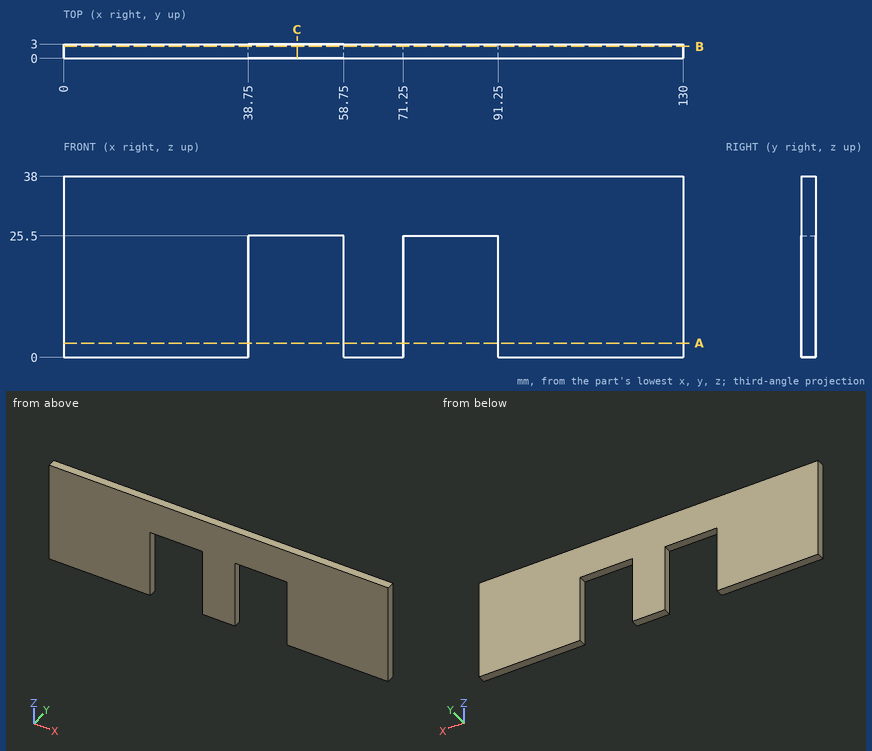
Study the drawing (mm; zero at the part's minimum x, y, z) and answer. Give positions to 0.01 mm unless a question says otherwise; leave off trailing zeros. Write each loop counter-clockwise with the first axis right and the second up, starting at its lowest first coordinate (ties: lowest second). Pieces come first, ordered by that corner, then holes. Notation, with made-up numbers: (61.25, 16.5) - (80.25, 16.5) arc R20 cw to (80.25, 49.5) - close; hole circle Ø10 at (54.25, 69). An arc over 180 degrees is marked (long way). Use CSV: the item, a comma, the result in double quotes. Start each with the question number.
(1) Find section A-A (z = 3). Give the vertices of the cut face in (x, y).
(2) Consider line 1 along X through (y, z) = (2.65, 11); line 2 along Z through (x, y) = (44, 1.65). Determine where each line is inside the solid, lowest interval first.
(3) Find section C-C (x = 49). Give the vertices of the cut face in (y, z).
(4) Find section B-B (y = 2.5). Give the vertices of the cut face in (x, z), plus the area to 3 significant figures.
(5) Given P1, Ø6, axis at x = 42, z = 11, coming from the +Y side, flat-ended and moving along its own axis, determine where the tip first touches the part or whether it passes through.
Findings below:
1,outline,"(0, 0) - (38.75, 0) - (38.75, 3) - (0, 3) - close; (58.75, 0) - (71.25, 0) - (71.25, 3) - (58.75, 3) - close; (91.25, 0) - (130, 0) - (130, 3) - (91.25, 3) - close"
2,line 1,"0 to 38.75, 58.75 to 71.25, 91.25 to 130"
2,line 2,"25.5 to 38"
3,outline,"(0, 25.5) - (3, 25.5) - (3, 38) - (0, 38) - close"
4,outline,"(0, 0) - (38.75, 0) - (38.75, 25.5) - (58.75, 25.5) - (58.75, 0) - (71.25, 0) - (71.25, 25.5) - (91.25, 25.5) - (91.25, 0) - (130, 0) - (130, 38) - (0, 38) - close"
4,area,"3,920 mm2"
5,P1,"through"
